Here's how the part is built. I have some questions about the finished solid (model axes, mm). A direction names the side the tool comes from. Coordinates: 2 decimals unless noted, no trailing zeros. Write each loop counter-clockwise with the first axis right and the second up, starting at its lowest first coordinate (ties: lowest second). Pieces come first, ordered by that corner, then holes. Notation, with made-up numbers: (66, 77.25) -> (102, 77.25) arc R21 ccw to (102, 115.25) -> close; hole circle Ø4 at (-14, -10). An arc over 180 degrees is marked (long way). Put each result on its own line as item: value.
```python
from build123d import *

# Parameters (mm, degrees)
BOSS_EXTRUDE1_DEPTH     = 450
CUT_EXTRUDE1_START      = -3
CUT_EXTRUDE1_DEPTH      = 444
SKETCH4_W               = 250
SKETCH4_H               = 144
CUT_EXTRUDE2_DEPTH      = 100
SKETCH5_R               = 112.5
CUT_EXTRUDE3_DEPTH      = 3
CUT_EXTRUDE5_DEPTH      = 553.268050859
CUT_EXTRUDE5_DEPTH_BACK = 553.268050859
SKETCH7_R               = 5
BOSS_EXTRUDE2_DEPTH     = 7
BOSS_EXTRUDE3_DEPTH     = 7
CUT_EXTRUDE7_DEPTH      = 702.783442381
CUT_EXTRUDE7_DEPTH_BACK = 702.783442381
SKETCH12_W              = 100
SKETCH12_H              = 147.055014966
BOSS_EXTRUDE4_DEPTH     = 3
SKETCH14_W              = 100
SKETCH14_H              = 147
BOSS_EXTRUDE5_DEPTH     = 3
SKETCH15_R              = 2
CUT_EXTRUDE8_DEPTH      = 3


with BuildPart() as part:
    # Sketch2 → Boss-Extrude1 (new body)
    with BuildSketch(Plane(origin=(0, 0, 0), x_dir=(0, 0, -1), z_dir=(1, 0, 0))):
        Polygon((-250, 0), (250, 0), (250, 150), (150, 150), (-50, 200), (-250, 100), align=None)
    extrude(amount=-BOSS_EXTRUDE1_DEPTH)

    # Sketch3 → Cut-Extrude1 (cut)
    with BuildSketch(Plane(origin=(0, 0, 0), x_dir=(0, 0, -1), z_dir=(1, 0, 0)).offset(CUT_EXTRUDE1_START)):
        Polygon((-247, 98.145898034), (-247, 3), (247, 3), (247, 147), (149.630683123, 147), (-49.650969671, 196.820413198), align=None)
    extrude(amount=-CUT_EXTRUDE1_DEPTH, mode=Mode.SUBTRACT)

    # Sketch4 → Cut-Extrude2 (cut)
    with BuildSketch(Plane(origin=(0, 0, -250), x_dir=(-1, 0, 0), z_dir=(0, 0, -1))):
        with Locations((225, 78)):
            Rectangle(SKETCH4_W, SKETCH4_H)
    extrude(amount=-CUT_EXTRUDE2_DEPTH, mode=Mode.SUBTRACT)

    # Sketch5 → Cut-Extrude3 (cut)
    with BuildSketch(Plane.XZ):
        with Locations(Location((-225, 0, 0), (0, 0, 270))):
            Circle(SKETCH5_R)
    extrude(amount=-CUT_EXTRUDE3_DEPTH, mode=Mode.SUBTRACT)

    # Sketch7 → Cut-Extrude5 (cut, two sides: drawn at the far end of the back side and taken through both)
    with BuildSketch(Plane(origin=(0, 0, 0), x_dir=(0, 0, -1), z_dir=(1, 0, 0)).offset(-CUT_EXTRUDE5_DEPTH_BACK)):
        with Locations((-130, 20)):
            Circle(SKETCH7_R)
        with Locations((-27, 20)):
            Circle(SKETCH7_R)
        with Locations((76, 20)):
            Circle(SKETCH7_R)
    extrude(amount=CUT_EXTRUDE5_DEPTH + CUT_EXTRUDE5_DEPTH_BACK, mode=Mode.SUBTRACT)

    # Sketch9 → Boss-Extrude2 (add)
    with BuildSketch(Plane(origin=(0, 0, 0), x_dir=(0, 0, -1), z_dir=(1, 0, 0))):
        Polygon((-250, 100), (250, 100), (250, 150), (150, 150), (-50, 200), align=None)
    extrude(amount=-BOSS_EXTRUDE2_DEPTH)

    # Sketch10 → Boss-Extrude3 (add)
    with BuildSketch(Plane.ZY.offset(450)):
        Polygon((250, 100), (50, 200), (-150, 150), (-250, 150), (-250, 100), align=None)
    extrude(amount=-BOSS_EXTRUDE3_DEPTH)

    # Sketch11 → Cut-Extrude7 (cut, two sides: drawn at the far end of the back side and taken through both)
    with BuildSketch(Plane.XY.offset(250).offset(-CUT_EXTRUDE7_DEPTH_BACK)):
        Polygon((0, 100), (0, 200), (-5, 200), align=None)
        Polygon((-450, 200), (-450, 100), (-445, 200), align=None)
    extrude(amount=CUT_EXTRUDE7_DEPTH + CUT_EXTRUDE7_DEPTH_BACK, mode=Mode.SUBTRACT)

    # Sketch12 → Boss-Extrude4 (add)
    with BuildSketch(Plane.ZY.offset(100)):
        with Locations((-200, 76.472492517)):
            Rectangle(SKETCH12_W, SKETCH12_H)
    extrude(amount=BOSS_EXTRUDE4_DEPTH)

    # Sketch14 → Boss-Extrude5 (add)
    with BuildSketch(Plane(origin=(-350, 0, 0), x_dir=(0, 0, -1), z_dir=(1, 0, 0))):
        with Locations((200, 76.5)):
            Rectangle(SKETCH14_W, SKETCH14_H)
    extrude(amount=BOSS_EXTRUDE5_DEPTH)

    # Sketch15 → Cut-Extrude8 (cut)
    with BuildSketch(Plane(origin=(0, 3, 0), x_dir=(1, 0, 0), z_dir=(0, 1, 0))):
        with Locations(Location((-400, 96, 0), (0, 0, 270))):
            Circle(SKETCH15_R)
        with Locations(Location((-400, 56, 0), (0, 0, 270))):
            Circle(SKETCH15_R)
        with Locations(Location((-400, -7, 0), (0, 0, 270))):
            Circle(SKETCH15_R)
        with Locations(Location((-400, -47, 0), (0, 0, 270))):
            Circle(SKETCH15_R)
        with Locations(Location((-400, -110, 0), (0, 0, 270))):
            Circle(SKETCH15_R)
        with Locations(Location((-400, -150, 0), (0, 0, 270))):
            Circle(SKETCH15_R)
        with Locations(Location((-50, -150, 0), (0, 0, 90))):
            Circle(SKETCH15_R)
        with Locations(Location((-50, -110, 0), (0, 0, 90))):
            Circle(SKETCH15_R)
        with Locations(Location((-50, -47, 0), (0, 0, 90))):
            Circle(SKETCH15_R)
        with Locations(Location((-50, -7, 0), (0, 0, 90))):
            Circle(SKETCH15_R)
        with Locations(Location((-50, 56, 0), (0, 0, 90))):
            Circle(SKETCH15_R)
        with Locations(Location((-50, 96, 0), (0, 0, 90))):
            Circle(SKETCH15_R)
    extrude(amount=-CUT_EXTRUDE8_DEPTH, mode=Mode.SUBTRACT)


solid = part.part
```
Item 1: Which directions (+Z, -Z, +X, -X, +Y, -Y) give clear straight access to the entire face, cutting with the end or side of a thin tool? Please do faces 4 (the flat face through (-52, 150, -201)), 5 (the flat face through (-221.892, 148.174, 146.944)), 6 (the cylindrical face through (-113.457, 1.479, 14.645)).
Output:
face 4: -Z, +X, -X, +Y
face 5: none
face 6: -Y
Item 2: Imagine slicing it at D-D on z = -37. Write out the boundary of the cut face in (x, y).
Output:
outline: (-450, 0) -> (-331.24, 0) -> (-331.24, 3) -> (-447, 3) -> (-447, 100) -> (-443, 100) -> (-443, 175.16) -> (-7, 175.16) -> (-7, 100) -> (-3, 100) -> (-3, 3) -> (-118.76, 3) -> (-118.76, 0) -> (0, 0) -> (0, 100) -> (-3.91, 178.25) -> (-446.09, 178.25) -> (-450, 100) -> close
Item 3: Imagine slicing it at C-C on x = -290. Write out the boundary of the cut face in (y, z).
Output:
outline: (0, -250) -> (6, -250) -> (6, -247) -> (3, -247) -> (3, -91.82) -> (0, -91.82) -> close; (0, 91.82) -> (3, 91.82) -> (3, 247) -> (98.15, 247) -> (196.82, 49.65) -> (147, -149.63) -> (147, -150) -> (150, -150) -> (200, 50) -> (100, 250) -> (0, 250) -> close
Item 4: For P1, Ø0.9, axis at x = -204, z = -248.5, coming from the +Y side; P2, Ø3, axis at x = -144, z = 191, coming from the +Y side; P3, Ø6, axis at x = -351, z = 44.5, coming from the +Y side (3 decimals); P4, Ø1.2, axis at x = -5.5, z = -64.5, coming from the -Y side, each with a flat end and sliding along its axis, tell me the tip position at first contact or that it passes through.
Output:
P1: stops at y = 6
P2: stops at y = 130.25
P3: stops at y = 199.375
P4: stops at y = 0
Item 5: Imagine slicing it at B-B on y = 185. Write out the boundary of the cut face in (x, z).
Output:
outline: (-445.75, -10) -> (-4.25, -10) -> (-4.25, 80) -> (-445.75, 80) -> close; hole (-443, 2.37) -> (-7, 2.37) -> (-7, 73.29) -> (-443, 73.29) -> close
Item 6: Imagine slicing it at A-A on x = -390. Write out the boundary of the cut face in (y, z).
Output:
outline: (0, -250) -> (150, -250) -> (150, -150) -> (200, 50) -> (100, 250) -> (0, 250) -> close; hole (3, -247) -> (147, -247) -> (147, -149.63) -> (196.82, 49.65) -> (98.15, 247) -> (3, 247) -> close
Item 7: If we mould it in two halves opening along X, with no side actions, what happens to faces 1 (the flat face through (-221.948, 171.561, -51.385)), 2 (the flat face through (-221.9, 150.7, 148.6)), 3 (the flat face through (-448.09, 138.19, -3.5))? For each: released by +X, released by -X, zero draft, split by the parting line, or undercut.
Output:
face 1: undercut
face 2: zero draft
face 3: released by -X
Item 8: Please list where these lines run through material, in increasing order: line 1 along Z through (x, y) = (-447.65, 20); line 2 along X through (y, z) = (0.7, 150); line 3 along X through (y, z) = (159.5, -24.5) (3 decimals). Write a range as from..to.
Output:
line 1: z = -250..-81, -71..22, 32..125, 135..250
line 2: x = -450..-402, -398..-52, -48..0
line 3: x = -447.025..-443, -7..-2.975
